Part model, mm, in its own coordinate system. Face numbers are marked on the shaded views. Give positions to 0.01 mm unless a question says otherwise; leave off trailing zeros. Write each loop counter-clockwise with the first axis right and the second up, starting at its lowest first coordinate (ties: lowest second). Pieces come first, ordered by that corner, then holes.
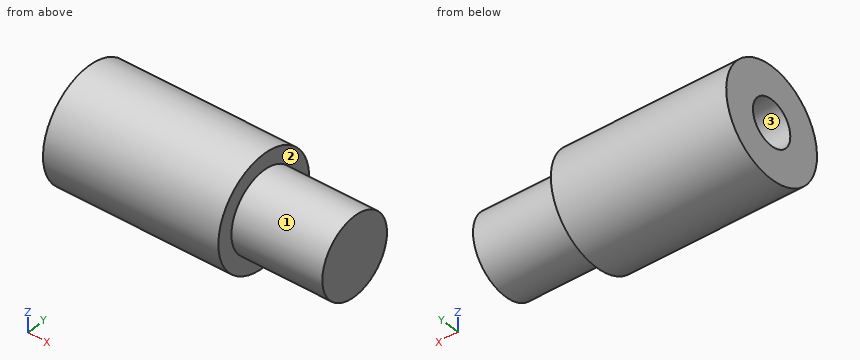
from build123d import *

# Parameters (mm, degrees)
SOCKET_1_SKETCH_W = 16.2
SOCKET_1_SKETCH_H = 3.175


with BuildPart() as part:
    # Conn_T4_MNPT Sketch → Conn_T4_MNPT (revolve)
    with BuildSketch(Plane.XY, mode=Mode.PRIVATE) as conn_t4_mnpt_sk:
        Polygon((12.7, 0), (12.7, 5.5), (0, 5.5), (0, 7.72), (-24.5, 7.72), (-24.5, 0), align=None)
    revolve(conn_t4_mnpt_sk.sketch.rotate(Axis((-1000, 0, 0), (1, 0, 0)), 90), axis=Axis((-1000, 0, 0), (1, 0, 0)))

    # Socket 1 Sketch → Socket 1 (revolve, cut)
    with BuildSketch(Plane.XY, mode=Mode.PRIVATE) as socket_1_sk:
        with Locations((-17.4, 1.5875)):
            Rectangle(SOCKET_1_SKETCH_W, SOCKET_1_SKETCH_H)
    revolve(socket_1_sk.sketch.rotate(Axis((-1000, 0, 0), (1, 0, 0)), 90), axis=Axis((-1000, 0, 0), (1, 0, 0)), mode=Mode.SUBTRACT)


solid = part.part
1) Mould opens along Z. For the marked faces 1, 2 and 3 say: +Z half, -Z half, draft (parallel to the pull), parting line (faces both ways), or undercut.
Check result:
face 1: parting line
face 2: draft
face 3: undercut
2) Saw through at A-A (z = 0). Write the cut outline in (x, y) (3 decimals).
Check result:
outline: (-24.5, -7.72) - (0, -7.72) - (0, -5.5) - (12.7, -5.5) - (12.7, 5.5) - (0, 5.5) - (0, 7.72) - (-24.5, 7.72) - (-24.5, 3.175) - (-9.3, 3.175) - (-9.3, -3.175) - (-24.5, -3.175) - close
3) Flat gauge pins, fed straight in: P1, Ø3, axis at x = -16.5, z = -3.5, coming from the +Y side; P2, Ø1.5, axis at x = -6, z = -4, coming from the +Y side; P3, Ø1.5, axis at x = -6, z = -1.5, coming from the +Y side. Where does each tip first touch, or does it go through?
Check result:
P1: stops at y = 7.46
P2: stops at y = 7
P3: stops at y = 7.68
4) Saw through at C-C (x = -20). Write the cut outline in (y, z) (3 decimals), and give its area (3 significant figures).
Check result:
outline: circle Ø15.44 at (0, 0); hole circle Ø6.35 at (0, 0)
area: 156 mm2
5) Drill centre lines: L1, parallel to X at y = 1, z = 2.25; L2, parallel to X at y = -3.25, z = 6.5; L3, parallel to Y at x = -20.5, z = 0 (3 decimals). Where is each one in solid material? Low to high.
Check result:
L1: x = -9.3 to 12.7
L2: x = -24.5 to 0
L3: y = -7.72 to -3.175, 3.175 to 7.72
6) Saw through at D-D (z = 4.5). Write the cut outline in (x, y).
Check result:
outline: (-24.5, -6.27) - (0, -6.27) - (0, -3.16) - (12.7, -3.16) - (12.7, 3.16) - (0, 3.16) - (0, 6.27) - (-24.5, 6.27) - close
